Autodesk Fusion 360 part; units mm, degrees
sketch "Sketch1" plane through (0, 0, 0) normal (0, 0, 1) x (1, 0, 0)
  line L0 (0, 0) -> (134, 0)
  line L1 (134, 0) -> (134, 50)
  line L2 (134, 50) -> (0, 50)
  line L3 (0, 50) -> (0, 0)
  circle A0 centre (7, 39) radius 1.55
  circle A1 centre (7, 11) radius 1.55
  circle A2 centre (127, 39) radius 1.55
  circle A3 centre (127, 11) radius 1.55
  line L4 (83.5, 21) -> (50.5, 21)
  line L5 (50.5, 21) -> (50.5, 29)
  line L6 (50.5, 29) -> (83.5, 29)
  line L7 (83.5, 29) -> (83.5, 21)
  line L8 (83.5, 21) -> (50.5, 29) construction
  line L9 (50.5, 21) -> (83.5, 29) construction
  line L10 (0, 25) -> (134, 25) construction
  circle A4 centre (40.5, 25) radius 1.55
  circle A5 centre (93.5, 25) radius 1.55
  line L11 (7, 11) -> (127, 11) construction
  line L12 (117, 9) -> (17, 9)
  line L13 (17, 9) -> (17, 13)
  line L14 (17, 13) -> (117, 13)
  line L15 (117, 13) -> (117, 9)
  line L16 (117, 9) -> (17, 13) construction
  line L17 (17, 9) -> (117, 13) construction
  line L18 (117, 41) -> (17, 41)
  line L19 (17, 41) -> (17, 37)
  line L20 (17, 37) -> (117, 37)
  line L21 (117, 37) -> (117, 41)
  line L22 (77, 9) -> (57, 9)
  line L23 (57, 9) -> (57, 13)
  line L24 (57, 13) -> (77, 13)
  line L25 (77, 13) -> (77, 9)
  line L26 (77, 9) -> (57, 13) construction
  line L27 (57, 9) -> (77, 13) construction
  point P0 (67, 25)
  point P1 (67, 11)
  point P2 (67, 11)
  dimension "d1" = 134
  dimension "d2" = 50
  dimension "d3" = 3.1
  dimension "d4" = 11
  dimension "d5" = 7
  dimension "d6" = 3.1
  dimension "d7" = 3.1
  dimension "d8" = 3.1
  dimension "d9" = 7
  dimension "d10" = 11
  dimension "d11" = 11
  dimension "d12" = 7
  dimension "d13" = 7
  dimension "d14" = 11
  dimension "d15" = 33
  dimension "d16" = 8
  dimension "d17" = 21
  dimension "d18" = 50.5
  dimension "d19" = 3.1
  dimension "d20" = 26.5
  dimension "d21" = 3.1
  dimension "d22" = 26.5
  dimension "d28" = 4
extrude "Extrude1" add sketch "Sketch1" along normal blind 1.5 contours L0 L1 L2 L3 | L12 L14 L15 L25 | L12 L14 L22 L23 L24 L25 | L12 L13 L14 L23 | L18 L19 L20 L21
extrude "Extrude2" add sketch "Sketch1" along normal blind 3 contours L12 L14 L15 L25 | L12 L13 L14 L23 | L18 L19 L20 L21
chamfer "Chamfer1" distance 1.5 angle 45 4 edges at (117, 11, 3) (117, 39, 3) (17, 39, 3) (17, 11, 3)
chamfer "Chamfer2" distance 1.5 angle 45 2 edges at (57, 11, 3) (77, 11, 3)
equation "d6 = d3"
equation "d7 = d3"
equation "d8 = d3"
equation "d9 = d5"
equation "d10 = d4"
equation "d11 = d4"
equation "d12 = d5"
equation "d13 = d5"
equation "d14 = d4"
equation "d19 = d3"
equation "d21 = d3"
equation "d22 = d20"
Work out the finished part from the listing and answer in its coordinate system (mm). Give positions to 0.01 mm unless a question says otherwise; leave off trailing zeros. Write each loop counter-clockwise with the first axis right and the second up, starting at its lowest first coordinate (ties: lowest second). Pieces come first, ordered by that corner, then holes. Notation, with made-up numbers: M 81.5,80.5 L 135.5,80.5 A31 ccw 135.5,109.5 Z; hole C 32,87.25 d10. An arc over 180 degrees is marked long. Answer as CSV lines item,"result".
Q1. A cutting plane is placed at B-B on x = 93.5. Write down the section's boundary in (y, z).
A:
outline,"M 0,0 L 23.45,0 L 23.45,1.5 L 13,1.5 L 13,3 L 9,3 L 9,1.5 L 0,1.5 Z; M 26.55,0 L 50,0 L 50,1.5 L 41,1.5 L 41,3 L 37,3 L 37,1.5 L 26.55,1.5 Z"
Q2. The mould has two halves that part along Y. Classify faces 1 (the cylindrical face through (41.33, 23.69, 0.74)), 2 (the flat face through (66, 39, 3)): +Y half, -Y half, draft (parallel to the pull), parting line (faces both ways), or undercut.
A:
face 1,"undercut"
face 2,"draft"
Q3. A cutting plane is placed at A-A on y = 25. Write down the section's boundary in (x, z), plus the area to 3 significant figures.
A:
outline,"M 0,0 L 38.95,0 L 38.95,1.5 L 0,1.5 Z; M 42.05,0 L 50.5,0 L 50.5,1.5 L 42.05,1.5 Z; M 83.5,0 L 91.95,0 L 91.95,1.5 L 83.5,1.5 Z; M 95.05,0 L 134,0 L 134,1.5 L 95.05,1.5 Z"
area,"142 mm²"
Q4. Find the intervals of material crossed by probe 1 along Y at (x, z) = (127, 1.05); probe 2 along Y at (x, z) = (96.5, 2.15); probe 3 along Y at (x, z) = (93.5, 0.45), in increasing order. Write a range as [from, to].
A:
probe 1,"y = [0, 9.45], [12.55, 37.45], [40.55, 50]"
probe 2,"y = [9, 13], [37, 41]"
probe 3,"y = [0, 23.45], [26.55, 50]"
Q5. A cutting plane is placed at C-C on x = 7. Write down the section's boundary in (y, z).
A:
outline,"M 0,0 L 9.45,0 L 9.45,1.5 L 0,1.5 Z; M 12.55,0 L 37.45,0 L 37.45,1.5 L 12.55,1.5 Z; M 40.55,0 L 50,0 L 50,1.5 L 40.55,1.5 Z"
Q6. A cutting plane is placed at D-D on z = 2.5. Write down the section's boundary in (x, y).
A:
outline,"M 18,9 L 56,9 L 56,13 L 18,13 Z; M 18,37 L 116,37 L 116,41 L 18,41 Z; M 78,9 L 116,9 L 116,13 L 78,13 Z"
Q7. Given P1, Ø15, axis at x = 43.5, y = 36, coming from the +Z side; P2, Ø8, axis at x = 90.5, y = 23.5, coming from the +Z side; P3, Ø0.5, axis at x = 106, z = 2, coming from the +Y side; P4, Ø0.8, axis at x = 79.5, z = 2, coming from the -Y side, each flat-ended and moving along its own axis, determine where each tip first touches the part or whether it passes through.
A:
P1,"stops at z = 3"
P2,"stops at z = 1.5"
P3,"stops at y = 41"
P4,"stops at y = 9"
